Work out the finished part from the listing and answer in its coordinate system (mm). Give positions to 0.01 mm unless a question says otherwise; leave off trailing zeros. Loops run counter-clockwise (first coordinate to the right, second up) from the corner with the lowest first, then second, coordinate; pieces in that order, holes last. Notation, with made-up numbers: (-18, 47) - (31, 47) arc R16 ccw to (31, 53) - close; hole circle Ø9 at (-1, -36.75). An arc over 180 degrees is marked (long way). One line per question, with ' | ' between items. Start each with the question number.
1. Section C-C (x = 59.5) is taken. Determine the outline of the cut face in (y, z).
2. Section D-D (y = 3) is taken. Determine the outline of the cut face in (x, z), plus the area to 3 significant figures.
3. This flat-tipped pin is pushed along its axis until it touches: pin 1 (4 mm diameter, centred on x = -41, y = 63.5, fed in from -Z). Where does it stop, or does it pass through?
4. Section B-B (x = -20) is taken. Determine the outline of the cut face in (y, z), plus the area to 3 significant figures.
5. Find the intervals of material crossed by line 1 (Z direction, x = 39, y = 21); line 2 (X direction, y = -43, z = 3.1), in increasing order.
6. Section A-A (y = 49.5) is taken. Determine the outline of the cut face in (x, z).
from build123d import *

# Parameters (mm, degrees)
SKETCH1_W           = 136
SKETCH1_H           = 174
BOSS_EXTRUDE1_DEPTH = 3
SKETCH2_W           = 124
SKETCH2_H           = 165
BOSS_EXTRUDE2_DEPTH = 0.25
SKETCH3_W           = 18.155382523
SKETCH3_H           = 24.50047974
BOSS_EXTRUDE3_DEPTH = 0.1


with BuildPart() as part:
    # Sketch1 → Boss-Extrude1 (new body)
    with BuildSketch(Plane.XY):
        Rectangle(SKETCH1_W, SKETCH1_H)
    extrude(amount=BOSS_EXTRUDE1_DEPTH)

    # Sketch2 → Boss-Extrude2 (add)
    with BuildSketch(Plane.XY.offset(3)):
        Rectangle(SKETCH2_W, SKETCH2_H)
    extrude(amount=BOSS_EXTRUDE2_DEPTH)

    # Sketch3 → Boss-Extrude3 (add)
    with BuildSketch(Plane(origin=(0, 0, 0), x_dir=(-1, 0, 0), z_dir=(0, 0, -1))):
        with Locations((-58.922308738, 4.333016158)):
            Rectangle(SKETCH3_W, SKETCH3_H)
    extrude(amount=BOSS_EXTRUDE3_DEPTH)


solid = part.part
Conclusion:
1) outline: (-87, 0) - (-7.92, 0) - (-7.92, -0.1) - (16.58, -0.1) - (16.58, 0) - (87, 0) - (87, 3) - (82.5, 3) - (82.5, 3.25) - (-82.5, 3.25) - (-82.5, 3) - (-87, 3) - close
2) outline: (-68, 0) - (49.84, 0) - (49.84, -0.1) - (68, -0.1) - (68, 3) - (62, 3) - (62, 3.25) - (-62, 3.25) - (-62, 3) - (-68, 3) - close | area: 441 mm²
3) pin 1: z = 0
4) outline: (-87, 0) - (87, 0) - (87, 3) - (82.5, 3) - (82.5, 3.25) - (-82.5, 3.25) - (-82.5, 3) - (-87, 3) - close | area: 563 mm²
5) line 1: 0 to 3.25 | line 2: -62 to 62
6) outline: (-68, 0) - (68, 0) - (68, 3) - (62, 3) - (62, 3.25) - (-62, 3.25) - (-62, 3) - (-68, 3) - close
